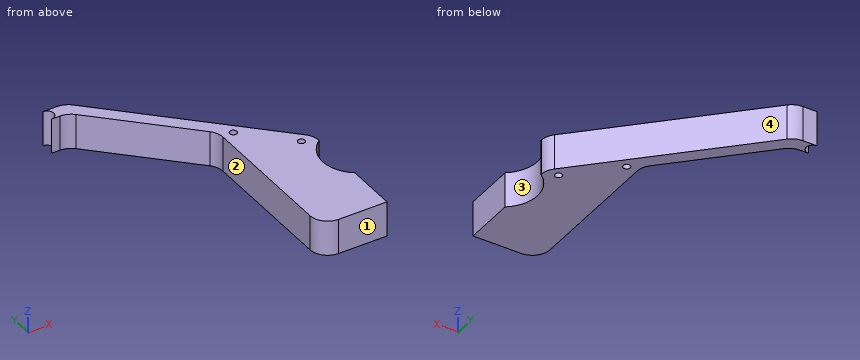
```python
from build123d import *

# Parameters (mm, degrees)
EXTRUDE_618_DEPTH   = 8
HOLE_WIZARD_M2_D    = 1.6
SKETCH_5_W          = 15
SKETCH_5_H          = 23
EXTRUDE_1905_DEPTH  = 8
FILLET_1_R          = 4
CUT_EXTRUDE_1_DEPTH = 60.03470161


with BuildPart() as part:
    # Эскиз1 → Extrude 618 (new body)
    with BuildSketch(Plane.XY):
        with BuildLine():
            Line((0.03033425, 5), (-14.96966575, 5))
            Line((-14.96966575, 5), (-14.96966575, 18.96966575))
            Line((-14.96966575, 18.96966575), (-36, 40))
            Line((-36, 40), (-39.64966575, 40))
            ThreePointArc((-39.64966575, 40), (-38.14966575, 41.5), (-39.64966575, 43))
            Line((-39.64966575, 43), (-34.757359313, 43))
            Line((-34.757359313, 43), (0.03033425, 8.212306438))
            Line((0.03033425, 8.212306438), (0.03033425, 5))
        make_face()
    extrude(amount=-EXTRUDE_618_DEPTH)

    # Крепление M2 (through all)
    with Locations(Plane.XY):
        with Locations((-2.96966575, 8), (-12.46966575, 17.5)):
            Hole(HOLE_WIZARD_M2_D / 2)

    # Эскиз5 → Extrude 1905 (add)
    with BuildSketch(Plane.XY):
        with Locations((-7.46966575, -6.5)):
            Rectangle(SKETCH_5_W, SKETCH_5_H)
    extrude(amount=-EXTRUDE_1905_DEPTH)

    # Скругление1
    fillet_1_edges = [part.edges().sort_by_distance(p)[0] for p in [
        (-14.96966575, 18.96966575, -4),
        (-36, 40, -4),
        (-34.757359313, 43, -4),
        (0.03033425, 8.212306438, -4),
        (-14.96966575, -18, -4),
    ]]
    fillet(fillet_1_edges, radius=FILLET_1_R)

    # Эскиз6 → Вырез-Вытянуть1 (cut, through all)
    with BuildSketch(Plane.XY):
        with BuildLine():
            Line((0.03033425, 6.437196595), (0.03033425, -6.437196595))
            ThreePointArc((0.03033425, -6.437196595), (-3.21966575, 0), (0.03033425, 6.437196595))
        make_face()
    extrude(amount=-CUT_EXTRUDE_1_DEPTH, mode=Mode.SUBTRACT)


solid = part.part
```
Geometry check sheet. Reference: the model listing, model coordinates, mm. Face numbers are marked on the shaded views. Give positions to 0.01 mm unless a question says otherwise; leave off trailing zeros. Write each loop counter-clockwise with the first axis right and the second up, starting at its lowest first coordinate (ties: lowest second). Pieces come first, ordered by that corner, then holes. Notation, with made-up numbers: (79.5, 67.5) - (111.5, 67.5) arc R16 ccw to (111.5, 95.5) - close; hole circle Ø2 at (-22.5, 25). An arc over 180 degrees is marked (long way). Use a Markdown table: item, result.
Q1. Section check C-C, the plane y = -13. Enter the section's corners in (x, z), then the cut area to 3 significant figures.
Computed:
| item | result |
|---|---|
| outline | (-14.97, -8) - (0.03, -8) - (0.03, 0) - (-14.97, 0) - close |
| area | 120 mm² |
Q2. Section check D-D, the plane x = -28.5. Enter the section's corners in (y, z), then the cut area to 3 significant figures.
Computed:
| item | result |
|---|---|
| outline | (32.5, -8) - (36.74, -8) - (36.74, 0) - (32.5, 0) - close |
| area | 33.9 mm² |
Q3. Go/stop test with flat-tipped pins: P1, Ø4, axis at y = 7.5, z = -5, coming from the -X side; P2, Ø2, axis at x = -38.5, z = -3.5, coming from the -Y side; P3, Ø1.5, axis at x = -27, z = -5.5, coming from the +Y side. Record where each tip stops, or that it passes through.
Computed:
| item | result |
|---|---|
| P1 | stops at x = -14.97 |
| P2 | stops at y = 40 |
| P3 | stops at y = 35.99 |
Q4. Section check B-B, the plane y = 8. Enter the section's corners in (x, z), then the cut area to 3 significant figures.
Computed:
| item | result |
|---|---|
| outline | (-14.97, -8) - (-3.77, -8) - (-3.77, 0) - (-14.97, 0) - close; (-2.17, -8) - (-0.24, -8) - (-0.24, 0) - (-2.17, 0) - close |
| area | 105 mm² |
Q5. Draft check along Y on the marked faces 1, 2, 3 and 4. Enter one of: pulls with the +Y half, pulls with the -Y half, needs draft (parallel to the pull), parting line crosses it, or undercut.
Computed:
| item | result |
|---|---|
| face 1 | pulls with the -Y half |
| face 2 | needs draft |
| face 3 | undercut |
| face 4 | pulls with the +Y half |
Q6. Section check A-A, the plane z = -6.75. Enter the section's corners in (x, y).
Computed:
| item | result |
|---|---|
| outline | (-39.65, 40) - (-37.66, 40) arc R4 cw to (-34.83, 38.83) - (-16.14, 20.14) arc R4 cw to (-14.97, 17.31) - (-14.97, -14) arc R4 ccw to (-10.97, -18) - (0.03, -18) - (0.03, -6.44) arc R8 cw to (0.03, 6.44) - (0.03, 6.56) arc R4 ccw to (-1.14, 9.38) - (-33.59, 41.83) arc R4 ccw to (-36.41, 43) - (-39.65, 43) arc R1.5 cw to start; hole circle Ø1.6 at (-12.47, 17.5); hole circle Ø1.6 at (-2.97, 8) |
Q7. Thickness scan on L1, parallel to Y at x = -13, z = -4.5; L2, parallel to Y at x = -8, z = -5.5; L3, parallel to X at y = 11.5, z = -1.75. Record the ranges inside material, lowest first. Write a range as [from, to].
Computed:
| item | result |
|---|---|
| L1 | y = [-17.45, 16.9], [18.1, 21.24] |
| L2 | y = [-18, 16.24] |
| L3 | x = [-14.97, -3.26] |
